The model under review builds one solid part; all positions refer to its coordinate system, in mm. Face numbers are marked on the shaded views. A direction names the side the tool comes from. Give positions to 0.01 mm unless a question says otherwise; leave off trailing zeros. Order: outer loops, then holes, each group sorted by start corner. A loop starts at its lowest first (then second) coordinate and runs counter-clockwise, first axis right, second up. Notation, with made-up numbers: (-15, 34.5) - (19, 34.5) arc R20 ccw to (19, 57.5) - close; hole circle Ø11 at (40, -34.75). An arc over 180 degrees is marked (long way). Put each result on its own line as item: value.
```python
from build123d import *

# Parameters (mm, degrees)
F0_W     = 12
F0_H     = 11.5
F0_H_2   = 4
F0_W_2   = 3.5
F0_H_3   = 8
F0_H_4   = 2.5
F0_W_3   = 2.5
F1_DEPTH = 1.6
F0_W_4   = 23
F0_H_5   = 7
F2_DEPTH = 7.5
F3_DEPTH = 5.6
F4_DEPTH = 9.6
F5_DEPTH = 14
F6_DEPTH = 10


with BuildPart() as f1:
    # F0 (on Top) → F1 (new body)
    with BuildSketch(Plane.XY):
        with BuildLine():
            Line((-11.5, 16), (-18.75, 16))
            ThreePointArc((-18.75, 16), (-19.2625631329, 14.7625631329), (-20.5, 14.25))
            Line((-20.5, 14.25), (-20.5, 1.5))
            Line((-20.5, 1.5), (-13.5, 1.5))
            Line((-13.5, 1.5), (-13.5, 4.5))
            Line((-13.5, 4.5), (-7.5, 4.5))
            Line((-7.5, 4.5), (-7.5, 1.5))
            Line((-7.5, 1.5), (-3, 1.5))
            Line((-3, 1.5), (-3, 4.5))
            Line((-3, 4.5), (3, 4.5))
            Line((3, 4.5), (3, 1.5))
            Line((3, 1.5), (7.5, 1.5))
            Line((7.5, 1.5), (7.5, 4.5))
            Line((7.5, 4.5), (13.5, 4.5))
            Line((13.5, 4.5), (13.5, 1.5))
            Line((13.5, 1.5), (20.5, 1.5))
            Line((20.5, 1.5), (20.5, 4))
            Line((20.5, 4), (18, 4))
            Line((18, 4), (18, 12))
            Line((18, 12), (20.5, 12))
            Line((20.5, 12), (20.5, 14.25))
            ThreePointArc((20.5, 14.25), (19.2625631329, 14.7625631329), (18.75, 16))
            Line((18.75, 16), (11.5, 16))
            Line((11.5, 16), (11.5, 9))
            Line((11.5, 9), (-11.5, 9))
            Line((-11.5, 9), (-11.5, 16))
        make_face()
        with BuildLine():
            ThreePointArc((-20.5, 14.25), (-21.7374368671, 17.2374368671), (-18.75, 16))
            Line((-18.75, 16), (-11.5, 16))
            Line((-11.5, 16), (-11.5, 20))
            Line((-11.5, 20), (-24, 20))
            Line((-24, 20), (-24, 1.5))
            Line((-24, 1.5), (-20.5, 1.5))
            Line((-20.5, 1.5), (-20.5, 14.25))
        make_face()
        with BuildLine():
            Line((11.5, 20), (11.5, 16))
            Line((11.5, 16), (18.75, 16))
            ThreePointArc((18.75, 16), (20.5, 17.75), (22.25, 16))
            ThreePointArc((22.25, 16), (21.7374368671, 14.7625631329), (20.5, 14.25))
            Line((20.5, 14.25), (20.5, 12))
            Line((20.5, 12), (24, 12))
            Line((24, 12), (24, 20))
            Line((24, 20), (11.5, 20))
        make_face()
        with BuildLine():
            Line((-13.5, 1.5), (-20.5, 1.5))
            Line((-20.5, 1.5), (-20.5, -14.4517312036))
            ThreePointArc((-20.5, -14.4517312036), (-18.7801368934, -14.5016722582), (-17.9343016893, -16))
            Line((-17.9343016893, -16), (-15.9493740648, -16))
            Line((-15.9493740648, -16), (-15.9493740648, -4.5))
            Line((-15.9493740648, -4.5), (-3.9493740648, -4.5))
            Line((-3.9493740648, -4.5), (-3.9493740648, -16))
            Line((-3.9493740648, -16), (18.75, -16))
            ThreePointArc((18.75, -16), (19.2625631329, -14.7625631329), (20.5, -14.25))
            Line((20.5, -14.25), (20.5, 1.5))
            Line((20.5, 1.5), (13.5, 1.5))
            Line((13.5, 1.5), (13.5, -1.5))
            Line((13.5, -1.5), (7.5, -1.5))
            Line((7.5, -1.5), (7.5, 1.5))
            Line((7.5, 1.5), (3, 1.5))
            Line((3, 1.5), (3, -1.5))
            Line((3, -1.5), (-3, -1.5))
            Line((-3, -1.5), (-3, 1.5))
            Line((-3, 1.5), (-7.5, 1.5))
            Line((-7.5, 1.5), (-7.5, -1.5))
            Line((-7.5, -1.5), (-13.5, -1.5))
            Line((-13.5, -1.5), (-13.5, 1.5))
        make_face()
        with BuildLine():
            Line((-20.5, -14.4517312036), (-20.5, 1.5))
            Line((-20.5, 1.5), (-24, 1.5))
            Line((-24, 1.5), (-24, -20))
            Line((-24, -20), (-15.9493740648, -20))
            Line((-15.9493740648, -20), (-15.9493740648, -16))
            Line((-15.9493740648, -16), (-17.9343016893, -16))
            ThreePointArc((-17.9343016893, -16), (-20.5884664851, -17.4983277418), (-20.5, -14.4517312036))
        make_face()
        with BuildLine():
            Line((18.75, -16), (-3.9493740648, -16))
            Line((-3.9493740648, -16), (-3.9493740648, -20))
            Line((-3.9493740648, -20), (24, -20))
            Line((24, -20), (24, 1.5))
            Line((24, 1.5), (20.5, 1.5))
            Line((20.5, 1.5), (20.5, -14.25))
            ThreePointArc((20.5, -14.25), (21.7374368671, -14.7625631329), (22.25, -16))
            ThreePointArc((22.25, -16), (20.5, -17.75), (18.75, -16))
        make_face()
        with Locations((-9.9493740648, -10.25)):
            Rectangle(F0_W, F0_H)
        with Locations((-9.9493740648, -18)):
            Rectangle(F0_W, F0_H_2)
        with Locations((22.25, 8)):
            Rectangle(F0_W_2, F0_H_3)
        with Locations((22.25, 2.75)):
            Rectangle(F0_W_2, F0_H_4)
        with Locations((19.25, 8)):
            Rectangle(F0_W_3, F0_H_3)
        with BuildLine():
            Line((-13.5, 4.5), (-13.5, 1.5))
            Line((-13.5, 1.5), (-12.25, 1.5))
            ThreePointArc((-12.25, 1.5), (-10.5, 3.25), (-8.75, 1.5))
            Line((-8.75, 1.5), (-7.5, 1.5))
            Line((-7.5, 1.5), (-7.5, 4.5))
            Line((-7.5, 4.5), (-13.5, 4.5))
        make_face()
        with BuildLine():
            Line((-3, 4.5), (-3, 1.5))
            Line((-3, 1.5), (-1.75, 1.5))
            ThreePointArc((-1.75, 1.5), (0, 3.25), (1.75, 1.5))
            Line((1.75, 1.5), (3, 1.5))
            Line((3, 1.5), (3, 4.5))
            Line((3, 4.5), (-3, 4.5))
        make_face()
        with BuildLine():
            Line((12.25, 1.5), (13.5, 1.5))
            Line((13.5, 1.5), (13.5, 4.5))
            Line((13.5, 4.5), (7.5, 4.5))
            Line((7.5, 4.5), (7.5, 1.5))
            Line((7.5, 1.5), (8.75, 1.5))
            ThreePointArc((8.75, 1.5), (10.5, 3.25), (12.25, 1.5))
        make_face()
        with BuildLine():
            ThreePointArc((-8.75, 1.5), (-10.5, 3.25), (-12.25, 1.5))
            Line((-12.25, 1.5), (-8.75, 1.5))
        make_face()
        with BuildLine():
            Line((-8.75, 1.5), (-12.25, 1.5))
            ThreePointArc((-12.25, 1.5), (-10.5, -0.25), (-8.75, 1.5))
        make_face()
        with BuildLine():
            Line((-12.25, 1.5), (-13.5, 1.5))
            Line((-13.5, 1.5), (-13.5, -1.5))
            Line((-13.5, -1.5), (-7.5, -1.5))
            Line((-7.5, -1.5), (-7.5, 1.5))
            Line((-7.5, 1.5), (-8.75, 1.5))
            ThreePointArc((-8.75, 1.5), (-10.5, -0.25), (-12.25, 1.5))
        make_face()
        with BuildLine():
            Line((-1.75, 1.5), (-3, 1.5))
            Line((-3, 1.5), (-3, -1.5))
            Line((-3, -1.5), (3, -1.5))
            Line((3, -1.5), (3, 1.5))
            Line((3, 1.5), (1.75, 1.5))
            ThreePointArc((1.75, 1.5), (0, -0.25), (-1.75, 1.5))
        make_face()
        with BuildLine():
            Line((1.75, 1.5), (-1.75, 1.5))
            ThreePointArc((-1.75, 1.5), (0, -0.25), (1.75, 1.5))
        make_face()
        with BuildLine():
            ThreePointArc((1.75, 1.5), (0, 3.25), (-1.75, 1.5))
            Line((-1.75, 1.5), (1.75, 1.5))
        make_face()
        with BuildLine():
            Line((8.75, 1.5), (12.25, 1.5))
            ThreePointArc((12.25, 1.5), (10.5, 3.25), (8.75, 1.5))
        make_face()
        with BuildLine():
            ThreePointArc((8.75, 1.5), (10.5, -0.25), (12.25, 1.5))
            Line((12.25, 1.5), (8.75, 1.5))
        make_face()
        with BuildLine():
            Line((13.5, -1.5), (13.5, 1.5))
            Line((13.5, 1.5), (12.25, 1.5))
            ThreePointArc((12.25, 1.5), (10.5, -0.25), (8.75, 1.5))
            Line((8.75, 1.5), (7.5, 1.5))
            Line((7.5, 1.5), (7.5, -1.5))
            Line((7.5, -1.5), (13.5, -1.5))
        make_face()
    extrude(amount=F1_DEPTH)

    # F0 (on Top) → F2 (join)
    with BuildSketch(Plane.XY):
        with Locations((0, 12.5)):
            Rectangle(F0_W_4, F0_H_5)
        with Locations((0, 18)):
            Rectangle(F0_W_4, F0_H_2)
    extrude(amount=F2_DEPTH)

    # F0 (on Top) → F3 (join)
    with BuildSketch(Plane.XY):
        with BuildLine():
            Line((-13.5, 4.5), (-13.5, 1.5))
            Line((-13.5, 1.5), (-12.25, 1.5))
            ThreePointArc((-12.25, 1.5), (-10.5, 3.25), (-8.75, 1.5))
            Line((-8.75, 1.5), (-7.5, 1.5))
            Line((-7.5, 1.5), (-7.5, 4.5))
            Line((-7.5, 4.5), (-13.5, 4.5))
        make_face()
        with BuildLine():
            Line((-12.25, 1.5), (-13.5, 1.5))
            Line((-13.5, 1.5), (-13.5, -1.5))
            Line((-13.5, -1.5), (-7.5, -1.5))
            Line((-7.5, -1.5), (-7.5, 1.5))
            Line((-7.5, 1.5), (-8.75, 1.5))
            ThreePointArc((-8.75, 1.5), (-10.5, -0.25), (-12.25, 1.5))
        make_face()
        with BuildLine():
            Line((-3, 4.5), (-3, 1.5))
            Line((-3, 1.5), (-1.75, 1.5))
            ThreePointArc((-1.75, 1.5), (0, 3.25), (1.75, 1.5))
            Line((1.75, 1.5), (3, 1.5))
            Line((3, 1.5), (3, 4.5))
            Line((3, 4.5), (-3, 4.5))
        make_face()
        with BuildLine():
            Line((-1.75, 1.5), (-3, 1.5))
            Line((-3, 1.5), (-3, -1.5))
            Line((-3, -1.5), (3, -1.5))
            Line((3, -1.5), (3, 1.5))
            Line((3, 1.5), (1.75, 1.5))
            ThreePointArc((1.75, 1.5), (0, -0.25), (-1.75, 1.5))
        make_face()
        with BuildLine():
            Line((12.25, 1.5), (13.5, 1.5))
            Line((13.5, 1.5), (13.5, 4.5))
            Line((13.5, 4.5), (7.5, 4.5))
            Line((7.5, 4.5), (7.5, 1.5))
            Line((7.5, 1.5), (8.75, 1.5))
            ThreePointArc((8.75, 1.5), (10.5, 3.25), (12.25, 1.5))
        make_face()
        with BuildLine():
            Line((13.5, -1.5), (13.5, 1.5))
            Line((13.5, 1.5), (12.25, 1.5))
            ThreePointArc((12.25, 1.5), (10.5, -0.25), (8.75, 1.5))
            Line((8.75, 1.5), (7.5, 1.5))
            Line((7.5, 1.5), (7.5, -1.5))
            Line((7.5, -1.5), (13.5, -1.5))
        make_face()
    extrude(amount=F3_DEPTH)

    # F0 (on Top) → F4 (join)
    with BuildSketch(Plane.XY):
        with BuildLine():
            ThreePointArc((1.75, 1.5), (0, 3.25), (-1.75, 1.5))
            Line((-1.75, 1.5), (1.75, 1.5))
        make_face()
        with BuildLine():
            Line((1.75, 1.5), (-1.75, 1.5))
            ThreePointArc((-1.75, 1.5), (0, -0.25), (1.75, 1.5))
        make_face()
        with BuildLine():
            ThreePointArc((-8.75, 1.5), (-10.5, 3.25), (-12.25, 1.5))
            Line((-12.25, 1.5), (-8.75, 1.5))
        make_face()
        with BuildLine():
            Line((-8.75, 1.5), (-12.25, 1.5))
            ThreePointArc((-12.25, 1.5), (-10.5, -0.25), (-8.75, 1.5))
        make_face()
        with BuildLine():
            Line((8.75, 1.5), (12.25, 1.5))
            ThreePointArc((12.25, 1.5), (10.5, 3.25), (8.75, 1.5))
        make_face()
        with BuildLine():
            ThreePointArc((8.75, 1.5), (10.5, -0.25), (12.25, 1.5))
            Line((12.25, 1.5), (8.75, 1.5))
        make_face()
    extrude(amount=F4_DEPTH)

    # F0 (on Top) → F5 (join)
    with BuildSketch(Plane.XY):
        with Locations((-9.9493740648, -10.25)):
            Rectangle(F0_W, F0_H)
        with Locations((-9.9493740648, -18)):
            Rectangle(F0_W, F0_H_2)
    extrude(amount=-F5_DEPTH)

    # F0 (on Top) → F6 (join)
    with BuildSketch(Plane.XY):
        with Locations((22.25, 8)):
            Rectangle(F0_W_2, F0_H_3)
        with Locations((19.25, 8)):
            Rectangle(F0_W_3, F0_H_3)
    extrude(amount=-F6_DEPTH)


solid = f1.part
```
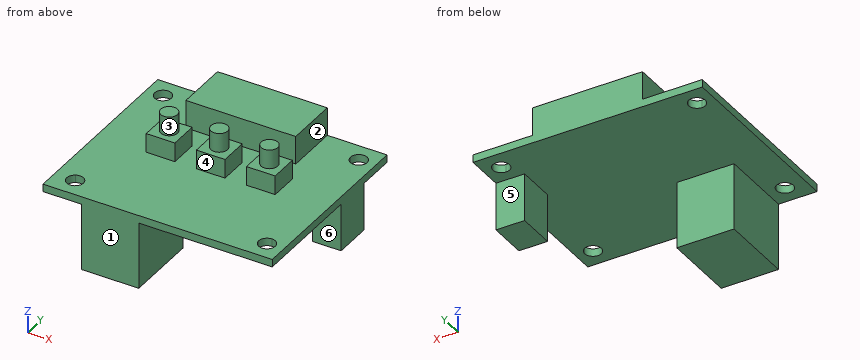
(1) Take a section at B-B, the plane y = 1.5. Write out the cut boundary in (x, z), then the cut area to 3 significant figures.
The answers:
outline: (-24, 0) - (24, 0) - (24, 1.6) - (13.5, 1.6) - (13.5, 5.6) - (12.25, 5.6) - (12.25, 9.6) - (8.75, 9.6) - (8.75, 5.6) - (7.5, 5.6) - (7.5, 1.6) - (3, 1.6) - (3, 5.6) - (1.75, 5.6) - (1.75, 9.6) - (-1.75, 9.6) - (-1.75, 5.6) - (-3, 5.6) - (-3, 1.6) - (-7.5, 1.6) - (-7.5, 5.6) - (-8.75, 5.6) - (-8.75, 9.6) - (-12.25, 9.6) - (-12.25, 5.6) - (-13.5, 5.6) - (-13.5, 1.6) - (-24, 1.6) - close
area: 191 mm^2
(2) The part is to be moulded in two halves that separate along Y. For the marked faces 1, 2 and 3, say which applies: pulls with the +Y half, pulls with the -Y half, needs draft (parallel to the pull), parting line crosses it, or undercut.
The answers:
face 1: pulls with the -Y half
face 2: needs draft
face 3: undercut
(3) Take a section at A-A, the plane z = 3.75. Write out the cut boundary in (x, y), then the cut area to 3 significant figures.
The answers:
outline: (-13.5, -1.5) - (-7.5, -1.5) - (-7.5, 4.5) - (-13.5, 4.5) - close; (-11.5, 9) - (11.5, 9) - (11.5, 20) - (-11.5, 20) - close; (-3, -1.5) - (3, -1.5) - (3, 4.5) - (-3, 4.5) - close; (7.5, -1.5) - (13.5, -1.5) - (13.5, 4.5) - (7.5, 4.5) - close
area: 361 mm^2
(4) Take a section at C-C, the plane x = 10.5. Write out the cut boundary in (y, z).
The answers:
outline: (-20, 0) - (20, 0) - (20, 7.5) - (9, 7.5) - (9, 1.6) - (4.5, 1.6) - (4.5, 5.6) - (3.25, 5.6) - (3.25, 9.6) - (-0.25, 9.6) - (-0.25, 5.6) - (-1.5, 5.6) - (-1.5, 1.6) - (-20, 1.6) - close
(5) For the marked faces 4, 5 and 6, list the 3-axis set-ups (+Z, -Z, +X, -X, +Y, -Y) from which the entire face can be reached by the end or side of a thin tool; tool diameter is ignored.
The answers:
face 4: +Z, +X, -X, -Y
face 5: -Z, +X, -X, +Y
face 6: -Z, +X, -X, -Y
(6) Wall thickness on L1, parallel to X at y = 16, z = 0.9; L2, parallel to X at y = -16, z = 1.1; L3, parallel to Y at x = -20.5, z = 0.7: over which ranges is each line inside the solid? List them lowest first.
The answers:
L1: -24 to -22.25, -18.75 to 18.75, 22.25 to 24
L2: -24 to -21.43, -17.93 to 18.75, 22.25 to 24
L3: -20 to -17.55, -14.45 to 14.25, 17.75 to 20
(7) Take a section at D-D, the plane z = -7.75. Write out the cut boundary in (x, y), then the cut area to 3 significant figures.
The answers:
outline: (-15.95, -20) - (-3.95, -20) - (-3.95, -4.5) - (-15.95, -4.5) - close; (18, 4) - (24, 4) - (24, 12) - (18, 12) - close
area: 234 mm^2
(8) Clearance check with flat-ended pins moving along their axes: pin 1 Ø1.5 at (x, z) = (19, -7.5) entering from -Y; pin 2 Ø4 at (x, y) = (-4, 8.5) entering from +Z; pin 3 Ø3 at (y, z) = (0, 3.5) entering from -X. State where each tip first meets the part, or that it passes through.
The answers:
pin 1: y = 4
pin 2: z = 7.5
pin 3: x = -13.5
